from build123d import *

# Parameters (mm, degrees)
EXTRUDE_1_DEPTH     = 28.9
SKETCH_2_R          = 1.2
CUT_EXTRUDE_1_DEPTH = 5


with BuildPart() as part:
    # 草图1 → 凸台-拉伸1 (new body)
    with BuildSketch(Plane.XY):
        with BuildLine():
            Line((-19.5, 8), (-20, 7.5))
            Line((-20, 7.5), (-20, 0.5))
            Line((-20, 0.5), (-19.5, 0))
            Line((-19.5, 0), (-14.5, 0))
            Line((-14.5, 0), (-14.5, 1.05))
            ThreePointArc((-14.5, 1.05), (-13.796309676, 1.277981519), (-13.36, 1.87530012))
            ThreePointArc((-13.36, 1.87530012), (-13.1, 2.25), (-13.36, 2.62469988))
            ThreePointArc((-13.36, 2.62469988), (-13.796309676, 3.222018481), (-14.5, 3.45))
            Line((-14.5, 3.45), (-14.5, 4.5))
            Line((-14.5, 4.5), (-5.5, 4.5))
            Line((-5.5, 4.5), (-5.5, 3.45))
            ThreePointArc((-5.5, 3.45), (-6.203690324, 3.222018481), (-6.64, 2.62469988))
            ThreePointArc((-6.64, 2.62469988), (-6.9, 2.25), (-6.64, 1.87530012))
            ThreePointArc((-6.64, 1.87530012), (-6.203690324, 1.277981519), (-5.5, 1.05))
            Line((-5.5, 1.05), (-5.5, 0))
            Line((-5.5, 0), (-0.5, 0))
            Line((-0.5, 0), (0, 0.5))
            Line((0, 0.5), (0, 7.5))
            Line((0, 7.5), (-0.5, 8))
            Line((-0.5, 8), (-19.5, 8))
        make_face()
    extrude(amount=-EXTRUDE_1_DEPTH)

    # 草图2 → 切除-拉伸1 (cut)
    with BuildSketch(Plane(origin=(0, 8, 0), x_dir=(1, 0, 0), z_dir=(0, 1, 0))):
        with Locations(Location((-17.5, 19.45, 0), (0, 0, 180))):
            Circle(SKETCH_2_R)
        with Locations(Location((-2.5, 19.45, 0), (0, 0, 180))):
            Circle(SKETCH_2_R)
        with Locations(Location((-2.5, 9.45, 0), (0, 0, 180))):
            Circle(SKETCH_2_R)
        with Locations(Location((-17.5, 9.45, 0), (0, 0, 180))):
            Circle(SKETCH_2_R)
    extrude(amount=-CUT_EXTRUDE_1_DEPTH, mode=Mode.SUBTRACT)


solid = part.part
Part model, mm, in its own coordinate system. A direction names the side the tool comes from. Coordinates: 2 decimals unless noted, no trailing zeros. Loops run counter-clockwise (first coordinate to the right, second up) from the corner with the lowest first, then second, coordinate; pieces in that order, holes last. Notation, with made-up numbers: (-24, 65) - (25, 65) arc R27 cw to (25, 87) - close; hole circle Ø4 at (25, -11.75). An arc over 180 degrees is marked (long way). Write each question's results on one line, items separated by ' | '. Start each with the question number.
Q1. Slice it at B-B on z = -23.5. Give the cut face in (x, y).
Q2. Slice it at C-C on x = -17.5. Give the cut face in (y, z).
Q3. Slice it at D-D on z = -9.45. Give the cut face in (x, y).
Q4. Which spindle directions (+Z, -Z, +X, -X, +Y, -Y) get a long thin tool onto all of the face, cutting with end or side? Do faces 1 (the flat face through (-3, 0, -14)), 2 (the flat face through (-14.5, 0.5, -14.2)), 3 (the flat face through (-10, 8, -14)), 4 (the flat face through (-10, 4.5, -14)), 5 (the flat face through (-2, 3, -9)). Say none if no direction does.
Q5. Slice it at A-A on y = 5.25. Give the cut face in (x, z), and give its area (3 significant figures).
Q6. Probe line 1 along Z through (x, y) = (-2.5, 7.5); line 2 along X through (y, z) = (4, -4.25); line 3 along X through (y, z) = (5.75, -20.25). List the from-to ranges inside material, lowest first.
Q7. Two-plate mould, pull along Y, no slides. Class faces 6 (the flat face through (0, 4, -14)), 7 (the cylindrical face through (-6.195, 3.228, -14.248)), 8 (the flat face through (-17, 3, -9)): +Y half, -Y half, draft (parallel to the pull), parting line (faces both ways), or undercut.
Q8. Drop flat-ended pins along their axis: pin 1 Ø1.2 at (x, z) = (-2, -9.5) entering from +Y; pin 2 Ø2.5 at (x, z) = (-11.5, -11) entering from -Y. Give the stop position or say it passes through.
Answer:
1) outline: (-20, 0.5) - (-19.5, 0) - (-14.5, 0) - (-14.5, 1.05) arc R1.2 ccw to (-13.36, 1.88) arc R0.4 ccw to (-13.36, 2.62) arc R1.2 ccw to (-14.5, 3.45) - (-14.5, 4.5) - (-5.5, 4.5) - (-5.5, 3.45) arc R1.2 ccw to (-6.64, 2.62) arc R0.4 ccw to (-6.64, 1.88) arc R1.2 ccw to (-5.5, 1.05) - (-5.5, 0) - (-0.5, 0) - (0, 0.5) - (0, 7.5) - (-0.5, 8) - (-19.5, 8) - (-20, 7.5) - close
2) outline: (0, -28.9) - (8, -28.9) - (8, -20.65) - (3, -20.65) - (3, -18.25) - (8, -18.25) - (8, -10.65) - (3, -10.65) - (3, -8.25) - (8, -8.25) - (8, 0) - (0, 0) - close
3) outline: (-20, 0.5) - (-19.5, 0) - (-14.5, 0) - (-14.5, 1.05) arc R1.2 ccw to (-13.36, 1.88) arc R0.4 ccw to (-13.36, 2.62) arc R1.2 ccw to (-14.5, 3.45) - (-14.5, 4.5) - (-5.5, 4.5) - (-5.5, 3.45) arc R1.2 ccw to (-6.64, 2.62) arc R0.4 ccw to (-6.64, 1.88) arc R1.2 ccw to (-5.5, 1.05) - (-5.5, 0) - (-0.5, 0) - (0, 0.5) - (0, 7.5) - (-0.5, 8) - (-1.3, 8) - (-1.3, 3) - (-3.7, 3) - (-3.7, 8) - (-16.3, 8) - (-16.3, 3) - (-18.7, 3) - (-18.7, 8) - (-19.5, 8) - (-20, 7.5) - close
4) face 1: +Z, -Z, +X, -X, -Y | face 2: +Z, -Z, -Y | face 3: +Z, -Z, +X, -X, +Y | face 4: +Z, -Z | face 5: +Y
5) outline: (-20, -28.9) - (0, -28.9) - (0, 0) - (-20, 0) - close; hole circle Ø2.4 at (-17.5, -19.45); hole circle Ø2.4 at (-17.5, -9.45); hole circle Ø2.4 at (-2.5, -19.45); hole circle Ø2.4 at (-2.5, -9.45) | area: 560 mm2
6) line 1: z = -28.9 to -20.65, -18.25 to -10.65, -8.25 to 0 | line 2: x = -20 to -14.5, -5.5 to 0 | line 3: x = -20 to -18.39, -16.61 to -3.39, -1.61 to 0
7) face 6: draft | face 7: undercut | face 8: +Y half
8) pin 1: stops at y = 3 | pin 2: stops at y = 4.5
